Autodesk Fusion 360 part; units mm, degrees
sketch "Sketch1" plane through (0, 0, 0) normal (0, 0, 1) x (1, 0, 0)
  line L0 (10.392, 2.2094) -> (17.5059, 5.2858)
  line L1 (13.949, 16.2125) -> (7.769, 5.9525)
  line L2 (18.4095, 14.7335) -> (18.4105, 6.6627)
  arc A0 (7.769, 5.9525) -> (11.3682, 2.6315) centre (9.9105, 4.6625) ccw
  circle A1 centre (9.9105, 4.6625) radius 1.75
  circle A2 centre (15.9105, 14.6625) radius 1.75
  arc A3 (17.5059, 5.2858) -> (18.4105, 6.6627) centre (16.9105, 6.6625) ccw
  arc A4 (18.4095, 14.5922) -> (13.6233, 15.6718) centre (15.9105, 14.6625) ccw
  dimension "d1" = 5
  dimension "d2" = 5
  dimension "d3" = 3
  dimension "d4" = 3.5
  dimension "d5" = 3.5
  dimension "d6" = 9.9105
  dimension "d7" = 4.6625
  dimension "d8" = 7.1139
  dimension "d9" = 3.0764
  dimension "d10" = 11.3682
  dimension "d11" = 8.0707
  dimension "d12" = 5.9525
  dimension "d13" = 16.2125
  dimension "d14" = 6.6627
extrude "Extrude1" add sketch "Sketch1" along normal blind 12 contours L0 L1 L2 A0 A3 A4
extrude "Extrude2" add sketch "Sketch1" along normal blind 16 from surface at -4 contours A1 | A2
For this review, take the finished solid that the model builds, in its own axes (mm). A direction names the side the tool comes from. Coordinates: 2 decimals unless noted, no trailing zeros. Loops run counter-clockwise (first coordinate to the right, second up) from the corner with the lowest first, then second, coordinate; pieces in that order, holes last. Notation, with made-up numbers: (-15.5, 39.5) -> (36.5, 39.5) arc R26 ccw to (36.5, 74.5) -> close; hole circle Ø9 at (71, 28). An arc over 180 degrees is marked (long way). Write each question's results on one line, items separated by ' | '.
Q1. Add section B-B, the plane x = 16.5. State the section outline as (y, z) points, then the cut area to 3 significant figures.
Taken from the geometry:
outline: (4.85, 0) -> (13.01, 0) -> (13.01, -4) -> (16.31, -4) -> (16.31, 0) -> (17.09, 0) -> (17.09, 12) -> (4.85, 12) -> close | area: 160 mm²
Q2. Add section C-C, the plane z = 2.5. State the section outline as (x, y) points, then the cut area to 3 significant figures.
Taken from the geometry:
outline: (7.77, 5.95) arc R2.5 ccw to (10.39, 2.21) -> (17.51, 5.29) arc R1.5 ccw to (18.41, 6.66) -> (18.41, 14.73) arc R2.5 ccw to (13.95, 16.21) -> close | area: 106 mm²
Q3. Add section A-A, the plane y = 16. State the section outline as (x, z) points, then the cut area to 3 significant figures.
Taken from the geometry:
outline: (13.82, 0) -> (14.78, 0) -> (14.78, -4) -> (17.04, -4) -> (17.04, 0) -> (18.02, 0) -> (18.02, 12) -> (13.82, 12) -> close | area: 59.4 mm²
Q4. Add section D-D, the plane z = -0.25. State the section outline as (x, y) points, then the cut area to 3 significant figures.
Taken from the geometry:
outline: circle Ø3.5 at (9.91, 4.66); circle Ø3.5 at (15.91, 14.66) | area: 19.2 mm²
Q5. Mouldability with a two-part tool opening along X and no side actions: class faces 3 (the cylindrical face through (18.17, 5.85, 5.92)), 4 (the flat face through (14, 10, 0)), 5 (the cylindrical face through (9.53, 6.37, -2.03)) as +X half, -X half, draft (parallel to the pull), parting line (faces both ways), or undercut.
Taken from the geometry:
face 3: +X half | face 4: draft | face 5: parting line
Q6. For pin 1 Ø5 at (x, z) = (10, 1.5) entering from +Y; pin 2 Ø2 at (x, z) = (14.5, 2.5) entering from +Y, all flat-tipped, find the tip position at first contact; note any pin that passes through.
Taken from the geometry:
pin 1: y = 13.81 | pin 2: y = 17.13
Q7. Machinability: for faces 1 (the flat face through (10, 5, -4)), 2 (the cylindrical face through (14.162, 14.586, -2.028)), which of the approach directions +Z, -Z, +X, -X, +Y, -Y give a long, thin tool a straight path to every point of the face, cutting with its end or side? Answer none if there is none.
Taken from the geometry:
face 1: -Z, +X, -X, +Y, -Y | face 2: -Z
Q8. To check wall thickness, follow line 1 along Z through (x, y) = (12.75, 6); line 2 along X through (y, z) = (4.75, 9.5); line 3 along X through (y, z) = (4, 9). State the ranges of each line that lie inside material, in increasing order. Write a range as [from, to].
Taken from the geometry:
line 1: [0, 12] | line 2: [7.41, 16.27] | line 3: [7.5, 14.53]
